Input: part model. Units: mm. Frame: model coordinates. Face numbers are marked on the shaded views. Give positions to 0.01 mm unless a question says otherwise; leave off trailing zeros. Loops run counter-clockwise (first coordinate to the right, second up) from the corner with the lowest first, then second, coordinate; pieces in that order, holes last. Notation, with made-up numbers: (-31, 48) -> (-12, 48) arc R19 cw to (-12, 56) -> close; hole circle Ø2 at (38, -18.5). An arc over 180 degrees is marked (long way). Answer as a JSON object with one key per item and string values.
```python
from build123d import *

# Parameters (mm, degrees)
F0_R     = 2
F1_DEPTH = 33.5
F2_R     = 1.308444
F3_DEPTH = 9.7
F4_W     = 5.071078
F4_H     = 2.256125
F4_R     = 1.013816
F5_DEPTH = 5


with BuildPart() as f1:
    # F0 (on Top) → F1 (new body)
    with BuildSketch(Plane.XY):
        Circle(F0_R)
    extrude(amount=F1_DEPTH)

    # F2 (on face) → F3 (join)
    with BuildSketch(Plane(origin=(0, 0, 0), x_dir=(1, 0, 0), z_dir=(0, 0, -1))):
        Circle(F2_R)
    extrude(amount=F3_DEPTH)

    # F4 (on Front) → F5 (join, symmetric)
    with BuildSketch(Plane.XZ):
        with Locations((0, 1.55916)):
            Rectangle(F4_W, F4_H)
        with Locations((0, 33.668082)):
            Circle(F4_R)
    extrude(amount=F5_DEPTH, both=True)


solid = f1.part
```
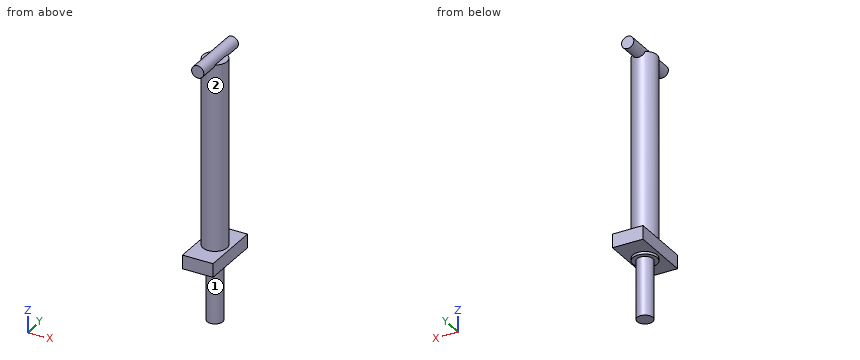
Q1. Section A-A, the plane y = -3.5. Return the cut outline in (x, z), then the cut area to 3 significant figures.
Evaluation:
{"outline": "(-2.54, 0.43) -> (2.54, 0.43) -> (2.54, 2.69) -> (-2.54, 2.69) -> close; circle Ø2.03 at (0, 33.67)", "area": "14.7 mm2"}
Q2. Draft query along Z for the marked faces 1 and 2. Return one class per face: +Z half, -Z half, draft (parallel to the pull), parting line (faces both ways), or undercut.
Evaluation:
{"face 1": "draft", "face 2": "undercut"}
Q3. Pin query (flat end, axial travel): pin 1 (0.5 mm diameter, centred on x = 1.5, y = -0.5, fed in from +Z); pin 2 (1.5 mm diameter, centred on x = 0.5, y = -2.5, fed in from -Z); pin 3 (1 mm diameter, centred on x = 2, z = 23.5, fed in from -Y). Return the tip coordinate at first contact, or that it passes through.
Evaluation:
{"pin 1": "stops at z = 33.5", "pin 2": "stops at z = 0", "pin 3": "stops at y = -1.32"}
Q4. Section B-B, the plane x = 0. Return the cut outline in (y, z).
Evaluation:
{"outline": "(-5, 0.43) -> (-2, 0.43) -> (-2, 0) -> (-1.31, 0) -> (-1.31, -9.7) -> (1.31, -9.7) -> (1.31, 0) -> (2, 0) -> (2, 0.43) -> (5, 0.43) -> (5, 2.69) -> (2, 2.69) -> (2, 32.65) -> (5, 32.65) -> (5, 34.68) -> (-5, 34.68) -> (-5, 32.65) -> (-2, 32.65) -> (-2, 2.69) -> (-5, 2.69) -> close"}
Q5. Section D-D, the plane z = 4.5. Return the cut outline in (x, y).
Evaluation:
{"outline": "circle Ø4 at (0, 0)"}
Q6. Ray query, line 1 along Z through (x, y) = (-1.75, -1.25); line 2 along X through (y, z) = (-1, 30); line 3 along Z through (x, y) = (-1.6, -0.25). Return the intervals inside material, ascending.
Evaluation:
{"line 1": "z = 0.43 to 2.69", "line 2": "x = -1.73 to 1.73", "line 3": "z = 0 to 33.5"}
Q7. Section C-C, the plane y = -0.75. Return the cut outline in (x, z).
Evaluation:
{"outline": "(-2.54, 0.43) -> (-1.85, 0.43) -> (-1.85, 0) -> (-1.07, 0) -> (-1.07, -9.7) -> (1.07, -9.7) -> (1.07, 0) -> (1.85, 0) -> (1.85, 0.43) -> (2.54, 0.43) -> (2.54, 2.69) -> (1.85, 2.69) -> (1.85, 33.5) -> (1, 33.5) arc R1.01 ccw (long way) to (-1, 33.5) -> (-1.85, 33.5) -> (-1.85, 2.69) -> (-2.54, 2.69) -> close"}
